```python
from build123d import *

# Parameters (mm, degrees)
SKETCH1_W           = 20
SKETCH1_H           = 20
BOSS_EXTRUDE1_DEPTH = 20
SKETCH2_W           = 45
SKETCH2_H           = 70
BOSS_EXTRUDE2_DEPTH = 8.3
CUT_EXTRUDE1_DEPTH  = 5.8
FILLET1_R           = 3.6
FILLET2_R           = 10
SKETCH5_R           = 3.9
CUT_EXTRUDE2_DEPTH  = 51.320373608
CUT_EXTRUDE3_REACH  = 49.302
SKETCH6_R           = 1.75
SKETCH13_W          = 20
SKETCH13_H          = 20
CUT_EXTRUDE9_DEPTH  = 20
SKETCH14_R          = 16.475
BOSS_EXTRUDE3_DEPTH = 7.6
SKETCH15_W          = 8.3
SKETCH15_H          = 45
CUT_EXTRUDE10_DEPTH = 15
FILLET3_R           = 23
CHAMFER1_SIZE       = 30
CHAMFER1_SIZE2      = 17.320508076
CHAMFER2_SIZE       = 30
CHAMFER2_SIZE2      = 17.320508076
SKETCH16_R          = 13.475
CUT_EXTRUDE11_DEPTH = 7.6
FILLET4_R           = 1


# Some blends are built 0.0001 mm under size
with BuildPart() as part:
    # Sketch1 → Boss-Extrude1 (new body)
    with BuildSketch(Plane(origin=(0, 0, 0), x_dir=(0, 0, -1), z_dir=(1, 0, 0))):
        Rectangle(SKETCH1_W, SKETCH1_H)
    extrude(amount=BOSS_EXTRUDE1_DEPTH)

    # Sketch2 → Boss-Extrude2 (add)
    with BuildSketch(Plane(origin=(20, 0, 0), x_dir=(0, 0, -1), z_dir=(1, 0, 0))):
        Rectangle(SKETCH2_W, SKETCH2_H)
    extrude(amount=BOSS_EXTRUDE2_DEPTH)

    # Sketch4 → Cut-Extrude1 (cut)
    with BuildSketch(Plane(origin=(28.3, 0, 0), x_dir=(0, 0, -1), z_dir=(1, 0, 0))):
        with BuildLine():
            Line((3.6, -28.55), (-3.6, -28.55))
            Line((-3.6, -28.55), (-3.6, -7.311805523))
            ThreePointArc((-3.6, -7.311805523), (0, 8.15), (3.6, -7.311805523))
            Line((3.6, -7.311805523), (3.6, -28.55))
        make_face()
    extrude(amount=-CUT_EXTRUDE1_DEPTH, mode=Mode.SUBTRACT)

    # Fillet1
    fillet1_edges = [part.edges().sort_by_distance(p)[0] for p in [
        (25.4, -28.55, 3.6),
        (25.4, -28.55, -3.6),
    ]]
    fillet(fillet1_edges, radius=FILLET1_R - 0.0001)  # a hair under: the kernel refuses the full size

    # Fillet2
    fillet2_edges = [part.edges().sort_by_distance(p)[0] for p in [
        (25.4, -7.311805523, 3.6),
        (25.4, -7.311805523, -3.6),
    ]]
    fillet(fillet2_edges, radius=FILLET2_R)

    # Sketch5 → Cut-Extrude2 (cut, through all)
    with BuildSketch(Plane.ZY):
        Circle(SKETCH5_R)
    extrude(amount=-CUT_EXTRUDE2_DEPTH, mode=Mode.SUBTRACT)

    # Sketch6 → Cut-Extrude3 (cut, up to next)
    with BuildSketch(Plane(origin=(22.5, 0, 0), x_dir=(0, 0, -1), z_dir=(1, 0, 0)), mode=Mode.PRIVATE) as cut_extrude3_sk1:
        with Locations((0, -20.6)):
            Circle(SKETCH6_R)
    cut_extrude3_tool1 = extrude(cut_extrude3_sk1.sketch, amount=-CUT_EXTRUDE3_REACH, mode=Mode.PRIVATE) & part.part
    # Sketch6 → Cut-Extrude3 (cut, up to next)
    with BuildSketch(Plane(origin=(22.5, 0, 0), x_dir=(0, 0, -1), z_dir=(1, 0, 0)), mode=Mode.PRIVATE) as cut_extrude3_sk2:
        with Locations((0, -9.35)):
            Circle(SKETCH6_R)
    cut_extrude3_tool2 = extrude(cut_extrude3_sk2.sketch, amount=-CUT_EXTRUDE3_REACH, mode=Mode.PRIVATE) & part.part
    add(cut_extrude3_tool1.solids().sort_by_distance((22.5, -20.6, 0))[0], mode=Mode.SUBTRACT)
    add(cut_extrude3_tool2.solids().sort_by_distance((22.5, -9.35, 0))[0], mode=Mode.SUBTRACT)

    # Sketch13 → Cut-Extrude9 (cut)
    with BuildSketch(Plane.ZY):
        Rectangle(SKETCH13_W, SKETCH13_H)
    extrude(amount=-CUT_EXTRUDE9_DEPTH, mode=Mode.SUBTRACT)

    # Sketch14 → Boss-Extrude3 (add)
    with BuildSketch(Plane.ZY.offset(-20)):
        with Locations(Location((0, 0, 0), (0, 0, 180))):
            Circle(SKETCH14_R)
    extrude(amount=BOSS_EXTRUDE3_DEPTH)

    # Sketch15 → Cut-Extrude10 (cut)
    with BuildSketch(Plane(origin=(0, 35, 0), x_dir=(1, 0, 0), z_dir=(0, 1, 0))):
        with Locations((24.15, 0)):
            Rectangle(SKETCH15_W, SKETCH15_H)
    extrude(amount=-CUT_EXTRUDE10_DEPTH, mode=Mode.SUBTRACT)

    # Fillet3
    # the kernel refuses this fillet: 23 mm, written as the material it takes off along each edge
    with BuildSketch(Plane(origin=(-37.5, 20, -22.5), x_dir=(0, -1, 0), z_dir=(1, 0, 0)), Plane(origin=(85.8, 20, 22.5), x_dir=(0, -1, 0), z_dir=(-1, 0, 0))) as fillet3_piece_1:
        with BuildLine():
            CenterArc((FILLET3_R, -FILLET3_R), FILLET3_R, 90, 90)
            Line((0, -FILLET3_R), (0, 0))
            Line((0, 0), (FILLET3_R, 0))
        make_face()
    extrude(amount=123.3, mode=Mode.SUBTRACT)

    # Chamfer1
    chamfer1_edges = [part.edges().sort_by_distance(p)[0] for p in [
        (24.15, -35, 22.5),
    ]]
    chamfer1_side = [part.faces().sort_by_distance(p)[0] for p in [
        (24.15, -19, 22.5),
    ]]
    chamfer(chamfer1_edges, length=CHAMFER1_SIZE, length2=CHAMFER1_SIZE2, reference=chamfer1_side[0])

    # Chamfer2
    chamfer2_edges = [part.edges().sort_by_distance(p)[0] for p in [
        (24.15, -35, -22.5),
    ]]
    chamfer2_side = [part.faces().sort_by_distance(p)[0] for p in [
        (24.15, -19, -22.5),
    ]]
    chamfer(chamfer2_edges, length=CHAMFER2_SIZE, length2=CHAMFER2_SIZE2, reference=chamfer2_side[0])

    # Sketch16 → Cut-Extrude11 (cut)
    with BuildSketch(Plane.ZY.offset(-12.4)):
        Circle(SKETCH16_R)
    extrude(amount=-CUT_EXTRUDE11_DEPTH, mode=Mode.SUBTRACT)

    # Fillet4
    fillet4_edges = [part.edges().sort_by_distance(p)[0] for p in [
        (20, 0, 16.475),
        (20, 0, -13.475),
    ]]
    fillet(fillet4_edges, radius=FILLET4_R)


solid = part.part
```
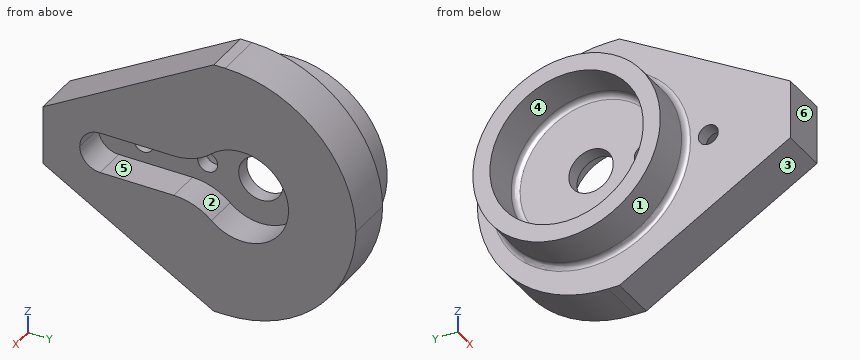
Here's how the part is built. I have some questions about the finished solid (model axes, mm). Face numbers are marked on the shaded views. A direction names the side the tool comes from. Coordinates: 2 decimals unless noted, no trailing zeros. Loops run counter-clockwise (first coordinate to the right, second up) from the corner with the lowest first, then second, coordinate; pieces in that order, holes last. Notation, with made-up numbers: (-33, 64.25) - (0, 64.25) arc R4 cw to (0, 68.25) - close; hole circle Ø9 at (78, 23). An arc over 180 degrees is marked (long way). Return JSON: item names as keys, results as strings. Group by question number.
Item 1: Will these pins go through, and if not, where does the flat tip stop? P1, Ø3, axis at x = 24, y = -21.5, coming from the -Z side; P2, Ø3, axis at x = 24.5, y = -16.5, coming from the +Z side; P3, Ø8, axis at x = 22, y = 4, coming from the +Z side.
Item 2: On a 3-axis mill with a long thin cutter (end or side, diameter ignored), from which of +Z, -Z, +X, -X, +Y, -Y can I reach the whole of each face in a straight line? I mean the marked faces 4, 5 and 6. Say none if no direction works.
Item 3: We'd pull the mould along Z, two halves only. Please class the marked faces 1, 2 and 3: +Z half, -Z half, draft (parallel to the pull), parting line (faces both ways), or undercut.
Item 4: If we section it at B-B on x = 14.5: Write out the boundary of the cut face in (y, z) (3 decimals).
Item 5: I need wall thicknesses on line 1 (Y direction, x = 15.75, z = 0) (3 decimals); line 2 (X direction, y = 3, z = 6.5); line 3 (Y direction, x = 14, z = -7.5). Which ranges of each line are inside material? Lowest first, please. Write a range as from..to.
Item 6: If we section it at D-D on y = -23.5: Write out the boundary of the cut face in (x, z).
Item 7: If we section it at C-C on z = -1: State how many separate pieces and enclosed holes the cut face has, and give its area (3 significant figures).
Calculated:
{
 "1": {"P1": "stops at z = -13.84", "P2": "stops at z = 16.73", "P3": "stops at z = 22.3"},
 "2": {"face 4": "-X", "face 5": "+X", "face 6": "+Z, -Z, +X, -X, -Y"},
 "3": {"face 1": "parting line", "face 2": "undercut", "face 3": "-Z half"},
 "4": {"outline": "circle Ø32.95 at (0, 0); hole circle Ø26.95 at (0, 0)"},
 "5": {"line 1": "y = -16.475..-13.475, 13.475..16.475", "line 2": "x = 20..22.5", "line 3": "y = -14.67..-11.19, 11.19..14.67"},
 "6": {"outline": "(20, -11.82) - (28.3, -11.82) - (28.3, -3.6) - (22.5, -3.6) - (22.5, 3.6) - (28.3, 3.6) - (28.3, 11.82) - (20, 11.82) - close"},
 "7": {"separate pieces": "4", "enclosed holes": "0", "area": "258 mm^2"}
}
